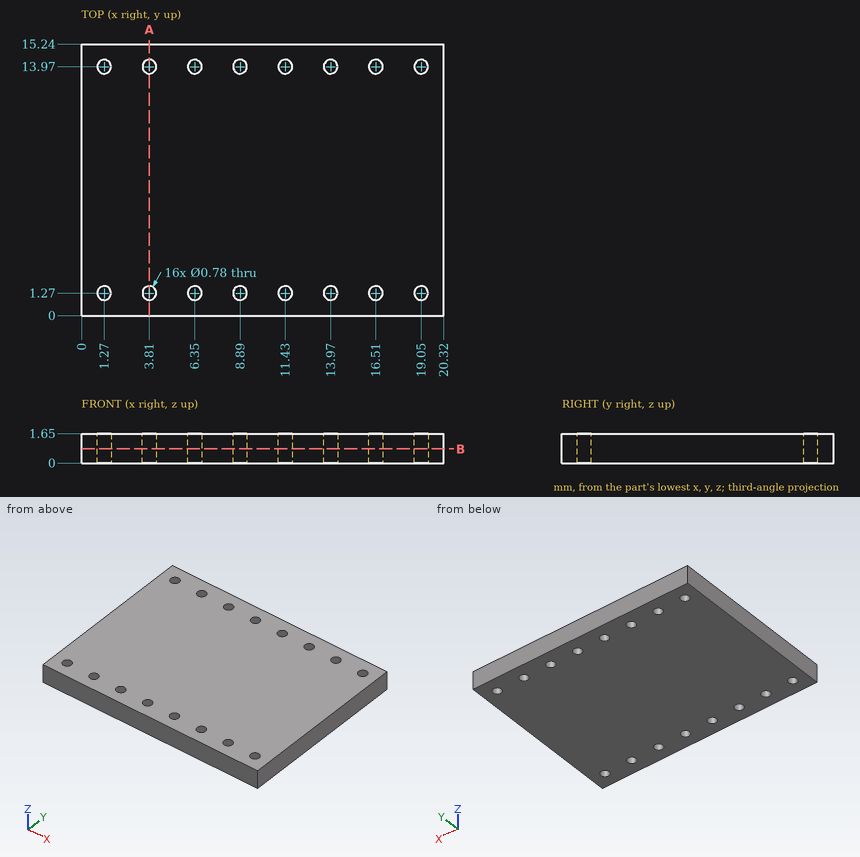
Here's the drawing with two shaded views (mm, measured from the low corner). I have some questions. Round coordinates to 2 decimals unless told otherwise and drop trailing zeros. Loops run counter-clockwise (first coordinate to the right, second up) from the corner with the lowest first, then second, coordinate; pieces in that order, holes last.
Item 1: Suppose I cut it at A-A, the plane x = 3.81. Write out the boundary of the cut face in (y, z), then the cut area to 3 significant figures.
Item 2: Please list where these lines run through material, in increasing order: L1, parallel to Y at x = 6.35, z = 0.7; L2, parallel to Y at x = 19.25, z = 1.3.
Item 3: Suppose I cut it at B-B, the plane z = 0.8. State how many separate pieces and enclosed holes the cut face has, then the cut area to 3 significant figures.
Reported:
1. outline: (0, 0) - (0.88, 0) - (0.88, 1.65) - (0, 1.65) - close; (1.66, 0) - (13.58, 0) - (13.58, 1.65) - (1.66, 1.65) - close; (14.36, 0) - (15.24, 0) - (15.24, 1.65) - (14.36, 1.65) - close
1. area: 22.6 mm2
2. L1: y = 0 to 0.88, 1.66 to 13.58, 14.36 to 15.24
2. L2: y = 0 to 0.94, 1.6 to 13.64, 14.3 to 15.24
3. separate pieces: 1
3. enclosed holes: 16
3. area: 302 mm2
